from build123d import *

# Parameters (mm, degrees)
CYLINDER001_R     = 4
CYLINDER001_DEPTH = 1.7
CYLINDER_R        = 8
CYLINDER_DEPTH    = 1.7
FILLET_R          = 0.3


with BuildPart() as cilindroint:
    # Cylinder001 → Cylinder001 (new body)
    with BuildSketch(Plane.XY):
        Circle(CYLINDER001_R)
    extrude(amount=CYLINDER001_DEPTH)


with BuildPart() as obj1:
    # Cylinder → Cylinder (new body)
    with BuildSketch(Plane.XY):
        Circle(CYLINDER_R)
    extrude(amount=CYLINDER_DEPTH)

    # Cut: cut cilindroInt
    add(cilindroint.part, mode=Mode.SUBTRACT)

    # Fillet
    fillet_edges = [obj1.edges().sort_by_distance(p)[0] for p in [
        (-8, 0, 1.7),
        (-8, 0, 0),
    ]]
    fillet(fillet_edges, radius=FILLET_R)


solid = obj1.part
Geometry: final body of the model. Coordinates: model frame, mm. Coordinates: 2 decimals unless noted, no trailing zeros. Order: outer loops, then holes, each group sorted by start corner. A loop starts at its lowest first (then second) coordinate and runs counter-clockwise, first axis right, second up. Notation, with made-up numbers: (51.25, -20) - (104.25, -20) arc R22 cw to (104.25, -13) - close; hole circle Ø7 at (20, 61). An arc over 180 degrees is marked (long way). Use one line per item in the form item = value.
1) Ray query, L1, parallel to Y at x = 0, z = 1; L2, parallel to Y at x = -3.25, z = 1.15; L3, parallel to X at y = -5, z = 1.3 (3 decimals). Return the intervals inside material, ascending.
Solutions:
L1 = -8 to -4, 4 to 8
L2 = -7.31 to -2.33, 2.33 to 7.31
L3 = -6.245 to 6.245
2) Section A-A (x = 0). Return loops of the section in (y, z), then the cut area to 3 significant figures.
Solutions:
outline = (-8, 0.3) arc R0.3 ccw to (-7.7, 0) - (-4, 0) - (-4, 1.7) - (-7.7, 1.7) arc R0.3 ccw to (-8, 1.4) - close; (4, 0) - (7.7, 0) arc R0.3 ccw to (8, 0.3) - (8, 1.4) arc R0.3 ccw to (7.7, 1.7) - (4, 1.7) - close
area = 13.5 mm^2
3) Mould query, pull axis Y, two halves, no side actions, for faces 1 (the face through (3, -3, 1.7)), 2 (the face through (-1.73, -7.81, 0.84)), 3 (the face through (-0.867, -3.905, 0.838)). Classes: +Y half, -Y half, draft (parallel to the pull), parting line (faces both ways), or undercut.
Solutions:
face_1 = draft
face_2 = parting line
face_3 = undercut
4) Section C-C (z = 0.85). Return loops of the section in (x, y).
Solutions:
outline = circle Ø16 at (0, 0); hole circle Ø8 at (0, 0)
